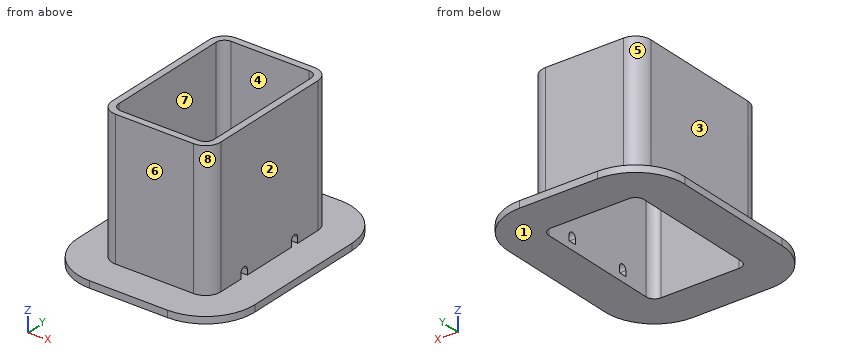
```python
from build123d import *

# Parameters (mm, degrees)
F1_DEPTH = 25.4
F2_DEPTH = 1.27
F4_DEPTH = 1.27


with BuildPart() as f1:
    # F0 (on Top) → F1 (new body)
    with BuildSketch(Plane.XY):
        with BuildLine():
            Line((10.16, -11.7475), (10.16, 11.7475))
            ThreePointArc((10.16, 11.7475), (9.323058, 13.768058), (7.3025, 14.605))
            Line((7.3025, 14.605), (-7.3025, 14.605))
            ThreePointArc((-7.3025, 14.605), (-9.323058, 13.768058), (-10.16, 11.7475))
            Line((-10.16, 11.7475), (-10.16, -11.7475))
            ThreePointArc((-10.16, -11.7475), (-9.323058, -13.768058), (-7.3025, -14.605))
            Line((-7.3025, -14.605), (7.3025, -14.605))
            ThreePointArc((7.3025, -14.605), (9.323058, -13.768058), (10.16, -11.7475))
        make_face()
        with BuildLine():
            Line((-7.3025, 13.335), (7.3025, 13.335))
            ThreePointArc((7.3025, 13.335), (8.425032, 12.870032), (8.89, 11.7475))
            Line((8.89, 11.7475), (8.89, -11.7475))
            ThreePointArc((8.89, -11.7475), (8.425032, -12.870032), (7.3025, -13.335))
            Line((7.3025, -13.335), (-7.3025, -13.335))
            ThreePointArc((-7.3025, -13.335), (-8.425032, -12.870032), (-8.89, -11.7475))
            Line((-8.89, -11.7475), (-8.89, 11.7475))
            ThreePointArc((-8.89, 11.7475), (-8.425032, 12.870032), (-7.3025, 13.335))
        make_face(mode=Mode.SUBTRACT)
    extrude(amount=F1_DEPTH)

    # F0 (on Top) + F1_face (on face) → F2 (join)
    with BuildSketch(Plane.XY):
        with BuildLine():
            Line((7.3025, 20.955), (-7.3025, 20.955))
            ThreePointArc((-7.3025, 20.955), (-13.813186, 18.258186), (-16.51, 11.7475))
            Line((-16.51, 11.7475), (-16.51, -11.7475))
            ThreePointArc((-16.51, -11.7475), (-13.813186, -18.258186), (-7.3025, -20.955))
            Line((-7.3025, -20.955), (7.3025, -20.955))
            ThreePointArc((7.3025, -20.955), (13.813186, -18.258186), (16.51, -11.7475))
            Line((16.51, -11.7475), (16.51, 11.7475))
            ThreePointArc((16.51, 11.7475), (13.813186, 18.258186), (7.3025, 20.955))
        make_face()
        with BuildLine():
            ThreePointArc((7.3025, 14.605), (9.323058, 13.768058), (10.16, 11.7475))
            Line((10.16, 11.7475), (10.16, -11.7475))
            ThreePointArc((10.16, -11.7475), (9.323058, -13.768058), (7.3025, -14.605))
            Line((7.3025, -14.605), (-7.3025, -14.605))
            ThreePointArc((-7.3025, -14.605), (-9.323058, -13.768058), (-10.16, -11.7475))
            Line((-10.16, -11.7475), (-10.16, 11.7475))
            ThreePointArc((-10.16, 11.7475), (-9.323058, 13.768058), (-7.3025, 14.605))
            Line((-7.3025, 14.605), (7.3025, 14.605))
        make_face(mode=Mode.SUBTRACT)
    with BuildSketch(Plane.XY.offset(25.4)):
        with BuildLine():
            Line((10.16, -11.7475), (10.16, 11.7475))
            ThreePointArc((10.16, 11.7475), (9.323058, 13.768058), (7.3025, 14.605))
            Line((7.3025, 14.605), (-7.3025, 14.605))
            ThreePointArc((-7.3025, 14.605), (-9.323058, 13.768058), (-10.16, 11.7475))
            Line((-10.16, 11.7475), (-10.16, -11.7475))
            ThreePointArc((-10.16, -11.7475), (-9.323058, -13.768058), (-7.3025, -14.605))
            Line((-7.3025, -14.605), (7.3025, -14.605))
            ThreePointArc((7.3025, -14.605), (9.323058, -13.768058), (10.16, -11.7475))
        make_face()
        with BuildLine():
            Line((-8.89, -11.7475), (-8.89, 11.7475))
            ThreePointArc((-8.89, 11.7475), (-8.425032, 12.870032), (-7.3025, 13.335))
            Line((-7.3025, 13.335), (7.3025, 13.335))
            ThreePointArc((7.3025, 13.335), (8.425032, 12.870032), (8.89, 11.7475))
            Line((8.89, 11.7475), (8.89, -11.7475))
            ThreePointArc((8.89, -11.7475), (8.425032, -12.870032), (7.3025, -13.335))
            Line((7.3025, -13.335), (-7.3025, -13.335))
            ThreePointArc((-7.3025, -13.335), (-8.425032, -12.870032), (-8.89, -11.7475))
        make_face(mode=Mode.SUBTRACT)
    extrude(amount=F2_DEPTH)

    # F3 (on face) → F4 (cut, through all)
    with BuildSketch(Plane.YZ.offset(10.16)):
        with BuildLine():
            Line((-6.858, 2.286), (-6.858, 1.27))
            Line((-6.858, 1.27), (-5.334, 1.27))
            Line((-5.334, 1.27), (-5.334, 2.286))
            ThreePointArc((-5.334, 2.286), (-6.096, 3.048), (-6.858, 2.286))
        make_face()
        with BuildLine():
            ThreePointArc((6.858, 2.286), (6.096, 3.048), (5.334, 2.286))
            Line((5.334, 2.286), (5.334, 1.27))
            Line((5.334, 1.27), (6.858, 1.27))
            Line((6.858, 1.27), (6.858, 2.286))
        make_face()
    extrude(amount=-F4_DEPTH, mode=Mode.SUBTRACT)


solid = f1.part
```
Read the model definition and answer for the solid it produces. Units are mm, in the model's axes. Face numbers are marked on the shaded views. A direction names the side the tool comes from. Coordinates: 2 decimals unless noted, no trailing zeros. Order: outer loops, then holes, each group sorted by start corner. A loop starts at its lowest first (then second) coordinate and runs counter-clockwise, first axis right, second up. Notation, with made-up numbers: (6, -18) - (35, -18) arc R13 cw to (35, -7) - close; hole circle Ø9 at (49.25, 50). An arc over 180 degrees is marked (long way). Answer as a JSON object with one key per item and string values. Group by question number.
Item 1: Section C-C (z = 11) is taken. Give the vertices of the cut face in (x, y) (1 decimal), plus the area to 3 significant figures.
Item 2: Section D-D (y = -17) is taken. Give the vertices of the cut face in (x, z).
Item 3: Section A-A (x = 0) is taken. Give the vertices of the cut face in (y, z) (3 decimals).
Item 4: Consider probe 1 along X at (y, z) = (-1.5, 10.25); probe 2 along Y at (x, z) = (-5, 15.5) (3 decimals); probe 3 along Z at (x, y) = (-4, -17). Determine where each line is inside the solid, lowest interval first. Write a range as from..to.
Item 5: Section B-B (y = -7.5) is taken. Give the vertices of the cut face in (x, z).
Item 6: Flat-ended cylindrical pins translate along their axes: P1, Ø6, axis at x = 2, z = 24, coming from the -Y side (3 decimals); P2, Ø0.8, axis at x = 9.5, z = 2, coming from the -Y side; P3, Ø4, axis at y = 3, z = 15, coming from the +X side. Find the tip coordinate at first contact, or state that the pin passes through.
Item 7: The mould has two halves that part along X. Classify the marked faces 1, 2, 3 and 4: +X half, -X half, draft (parallel to the pull), parting line (faces both ways), or undercut.
Item 8: A tool of negligible diameter and unlimited length cuts with its end or side. For the marked faces 5, 6, 7 and 8, from which of +Z, -Z, +X, -X, +Y, -Y can it reach the whole face along a straight path? Write none if from no direction.
Results are:
{
 "1": {"outline": "(-10.2, -11.7) arc R2.9 ccw to (-7.3, -14.6) - (7.3, -14.6) arc R2.9 ccw to (10.2, -11.7) - (10.2, 11.7) arc R2.9 ccw to (7.3, 14.6) - (-7.3, 14.6) arc R2.9 ccw to (-10.2, 11.7) - close; hole (-8.9, -11.7) arc R1.6 ccw to (-7.3, -13.3) - (7.3, -13.3) arc R1.6 ccw to (8.9, -11.7) - (8.9, 11.7) arc R1.6 ccw to (7.3, 13.3) - (-7.3, 13.3) arc R1.6 ccw to (-8.9, 11.7) - close", "area": "115 mm^2"},
 "2": {"outline": "(-14.86, 0) - (14.86, 0) - (14.86, 1.27) - (-14.86, 1.27) - close"},
 "3": {"outline": "(-20.955, 0) - (-13.335, 0) - (-13.335, 26.67) - (-14.605, 26.67) - (-14.605, 1.27) - (-20.955, 1.27) - close; (13.335, 0) - (20.955, 0) - (20.955, 1.27) - (14.605, 1.27) - (14.605, 26.67) - (13.335, 26.67) - close"},
 "4": {"probe 1": "x = -10.16..-8.89, 8.89..10.16", "probe 2": "y = -14.605..-13.335, 13.335..14.605", "probe 3": "z = 0..1.27"},
 "5": {"outline": "(-16.51, 0) - (-8.89, 0) - (-8.89, 26.67) - (-10.16, 26.67) - (-10.16, 1.27) - (-16.51, 1.27) - close; (8.89, 0) - (16.51, 0) - (16.51, 1.27) - (10.16, 1.27) - (10.16, 26.67) - (8.89, 26.67) - close"},
 "6": {"P1": "stops at y = -14.605", "P2": "stops at y = -13.97", "P3": "stops at x = 10.16"},
 "7": {"face 1": "draft", "face 2": "+X half", "face 3": "-X half", "face 4": "undercut"},
 "8": {"face 5": "+Z, -X, +Y", "face 6": "+Z, +X, -X, -Y", "face 7": "+Z, -Z", "face 8": "+Z, +X, -Y"}
}
